Input: part model. Units: mm. Frame: model coordinates. Face numbers are marked on the shaded views. A direction names the side the tool comes from. Give positions to 0.01 mm unless a question says otherwise; leave off trailing zeros. Order: outer loops, then holes, each group sorted by start corner. A loop starts at its lowest first (then second) coordinate and runs counter-clockwise, first axis right, second up. Notation, with made-up numbers: M -22.75,-36 L -6.75,-36 A16 ccw -6.75,-6 Z; hole C -19,14.25 d3. An arc over 180 degrees is marked long. Use a Markdown table: item, result.
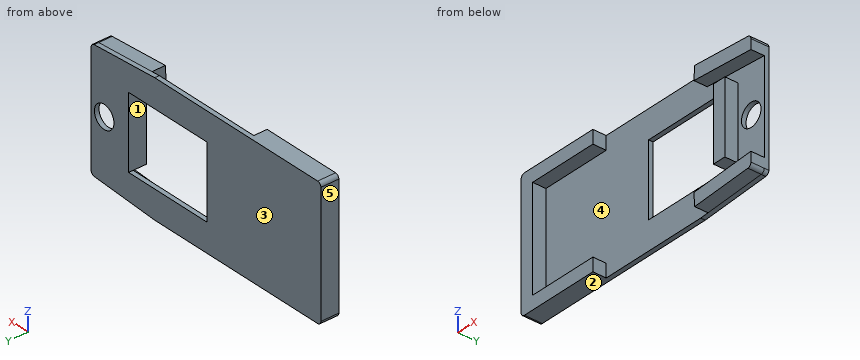
from build123d import *

# Parameters (mm, degrees)
SKETCH1_R           = 3
SKETCH1_W           = 24
SKETCH1_H           = 19
BOSS_EXTRUDE1_DEPTH = 1.2
SKETCH2_W           = 3.5
SKETCH2_H           = 19
BOSS_EXTRUDE2_DEPTH = 3.5
FILLET1_R           = 1


with BuildPart() as part:
    # Sketch1 → Boss-Extrude1 (new body)
    with BuildSketch(Plane(origin=(0, 0, 0), x_dir=(1, 0, 0), z_dir=(0, 1, 0))):
        Polygon((51, 33.8), (70.5, 32.475), (70.5, 1.325), (51, 0), (0, 0), (0, 33.8), align=None)
        with Locations(Location((66.5, 16.9, 0), (0, 0, 270))):
            Circle(SKETCH1_R, mode=Mode.SUBTRACT)
        with Locations((47, 16.9)):
            Rectangle(SKETCH1_W, SKETCH1_H, mode=Mode.SUBTRACT)
    extrude(amount=BOSS_EXTRUDE1_DEPTH)

    # Sketch2 → Boss-Extrude2 (add)
    with BuildSketch(Plane.XZ):
        Polygon((0, 0), (22, 0), (22, -3.5), (3.5, -3.5), (3.5, -30.3), (22, -30.3), (22, -33.8), (4.40507534, -33.8), (0, -33.8), (0, -3.5), align=None)
        Polygon((53.236727535, -0.151982768), (70.5, -1.325), (70.5, -4.825), (53, -3.635897436), align=None)
        Polygon((70.5, -32.475), (53.236727535, -33.648017232), (53, -30.164102564), (70.5, -28.975), align=None)
        with Locations((60.75, -16.9)):
            Rectangle(SKETCH2_W, SKETCH2_H)
    extrude(amount=BOSS_EXTRUDE2_DEPTH)

    # Fillet1
    fillet1_edges = [part.edges().sort_by_distance(p)[0] for p in [
        (0, -1.15, -33.8),
        (70.5, -1.15, -32.475),
        (70.5, -1.15, -1.325),
        (0, -1.15, 0),
    ]]
    fillet(fillet1_edges, radius=FILLET1_R)


solid = part.part
1) Cut plane D-D on z = -23. Return loops of the section in (x, y), and give its area (3 significant figures).
Response values:
| item | result |
|---|---|
| outline | M 0,-3.5 L 3.5,-3.5 L 3.5,0 L 35,0 L 35,1.2 L 0,1.2 Z; M 59,-3.5 L 62.5,-3.5 L 62.5,0 L 70.5,0 L 70.5,1.2 L 59,1.2 Z |
| area | 80.3 mm² |
2) Mould query, pull axis X, two halves, no side actions, for the marked faces 3, 4 and 5. Classes: released by +X, released by -X, zero draft, split by the parting line, or undercut.
Response values:
| item | result |
|---|---|
| face 3 | zero draft |
| face 4 | undercut |
| face 5 | released by -X |
3) First-contact query: pin 1 Ø1 at (y, z) = (-2.5, -10.5) entering from +X; pin 2 Ø17 at (x, z) = (43, -20) entering from -Y; pin 3 Ø1.3 at (x, y) = (51.5, 0.5) entering from +Z; pin 4 Ø3.5 at (x, z) = (66.5, -16.9) entering from +Y. Flat tips, straight axial feed; report the tip coordinate or a pass-through.
Response values:
| item | result |
|---|---|
| pin 1 | stops at x = 62.5 |
| pin 2 | stops at y = 0 |
| pin 3 | stops at z = 0 |
| pin 4 | passes through |
4) Cut plane A-A on x = 41.5. Return loops of the section in (y, z), and give its area (3 significant figures).
Response values:
| item | result |
|---|---|
| outline | M 0,-33.8 L 1.2,-33.8 L 1.2,-26.4 L 0,-26.4 Z; M 0,-7.4 L 1.2,-7.4 L 1.2,0 L 0,0 Z |
| area | 17.8 mm² |
5) Cut plane C-C on y = -1.9. Return loops of the section in (x, z) (3 decimals), and give its area (3 significant figures).
Response values:
| item | result |
|---|---|
| outline | M 0,-32.8 A1 ccw 1,-33.8 L 22,-33.8 L 22,-30.3 L 3.5,-30.3 L 3.5,-3.5 L 22,-3.5 L 22,0 L 1,0 A1 ccw 0,-1 Z; M 53,-30.164 L 53.237,-33.648 L 69.568,-32.538 A1 ccw 70.5,-31.541 L 70.5,-28.975 Z; M 53,-3.636 L 70.5,-4.825 L 70.5,-2.259 A1 ccw 69.568,-1.262 L 53.237,-0.152 Z; M 59,-26.4 L 62.5,-26.4 L 62.5,-7.4 L 59,-7.4 Z |
| area | 435 mm² |
6) Reachability of the marked faces 1 and 2 from +Z, -Z, +X, -X, +Y, -Y: full face, straight path, thin tool, end or side. Return the list, or none.
Response values:
| item | result |
|---|---|
| face 1 | +Y, -Y |
| face 2 | -Z, +X, -X, +Y, -Y |
7) Cut plane B-B on z = -16.9. Return loops of the section in (x, y).
Response values:
| item | result |
|---|---|
| outline | M 0,-3.5 L 3.5,-3.5 L 3.5,0 L 35,0 L 35,1.2 L 0,1.2 Z; M 59,-3.5 L 62.5,-3.5 L 62.5,0 L 63.5,0 L 63.5,1.2 L 59,1.2 Z; M 69.5,0 L 70.5,0 L 70.5,1.2 L 69.5,1.2 Z |
8) Material intervals for line 1 (X direction, y = 0.55, z = -16.9); line 2 (Z direction, x = 17, y = -1.45); line 3 (X direction, y = -1.4, z = -18), sorted ascending. Write a range as from..to.
Response values:
| item | result |
|---|---|
| line 1 | x = 0..35, 59..63.5, 69.5..70.5 |
| line 2 | z = -33.8..-30.3, -3.5..0 |
| line 3 | x = 0..3.5, 59..62.5 |
